Autodesk Inventor part; units mm, degrees
ref_plane "YZ Plane" through (0, 0, 0) normal (1, 0, 0) x (0, 1, 0)
ref_plane "XZ Plane" through (0, 0, 0) normal (0, 1, 0) x (-1, 0, 0)
ref_plane "XY Plane" through (0, 0, 0) normal (0, 0, 1) x (1, 0, 0)
sketch "Sketch1" plane through (0, 0, 0) normal (0, 1, 0) x (-1, 0, 0)
  circle A0 centre (0, 0) radius 57.785
  circle A1 centre (0, 0) radius 148.0058
  line L0 (0, 0) -> (-122.3635, 70.6466) construction
  line L1 (0, 0) -> (141.2932, 0) construction
  line L2 (-122.3635, 70.6466) -> (0, 0) construction
  line L3 (0, 0) -> (-128.1768, -74.0029) construction
  circle A2 centre (0, 0) radius 148.0058 construction
  line L4 (0, 0) -> (148.0058, 0) construction
  circle A3 centre (0, 0) radius 137.541 construction
  circle A4 centre (-119.114, -68.7705) radius 3.175
  circle A5 centre (0, -137.541) radius 3.175
  circle A6 centre (119.114, -68.7705) radius 3.175
  circle A7 centre (119.114, 68.7705) radius 3.175
  circle A8 centre (0, 137.541) radius 3.175
  circle A9 centre (-119.114, 68.7705) radius 3.175
  dimension "d22" = 275.082
  dimension "d16" = 115.57
  dimension "d17" = 296.0116
  dimension "d20" = 150
  dimension "d21" = 150
  dimension "d23" = 6.35
  dimension "d24" = 360
extrude "Extrusion1" add sketch "Sketch1" along normal blind 12.7
sketch "Sketch2" plane through (0, 12.7, 0) normal (0, 1, 0) x (1, 0, 0)
  circle A0 centre (0, 0) radius 123.4694 construction
  line L0 (-21.15, -84.9341) -> (-21.15, -115.9341) construction
  line L1 (15.5, -121.5841) -> (-15.5, -121.5841) construction
  line L2 (21.15, -115.9341) -> (21.15, -84.9341) construction
  line L3 (-15.5, -79.2841) -> (15.5, -79.2841) construction
  line L4 (15.5, -79.2841) -> (21.15, -84.9341) construction
  line L5 (21.15, -115.9341) -> (15.5, -121.5841) construction
  line L6 (-15.5, -121.5841) -> (-21.15, -115.9341) construction
  line L7 (-21.15, -84.9341) -> (-15.5, -79.2841) construction
  line L8 (-15.5, -115.9341) -> (15.5, -115.9341) construction
  line L9 (15.5, -115.9341) -> (15.5, -84.9341) construction
  line L10 (15.5, -84.9341) -> (-15.5, -84.9341) construction
  line L11 (-15.5, -84.9341) -> (-15.5, -115.9341) construction
  line L12 (-15.5, -115.9341) -> (15.5, -84.9341) construction
  line L13 (15.5, -115.9341) -> (-15.5, -84.9341) construction
  circle A1 centre (15.5, -84.9341) radius 1.5
  circle A2 centre (15.5, -115.9341) radius 1.5
  circle A3 centre (-15.5, -115.9341) radius 1.5
  circle A4 centre (-15.5, -84.9341) radius 1.5
  circle A5 centre (0, -100.4341) radius 11.049
  circle A6 centre (0, -100.4341) radius 22.9616 construction
  dimension "d27" = 246.9388
  dimension "d32" = 3
  dimension "d33" = 3
  dimension "d34" = 3
  dimension "d35" = 22.098
  dimension "d44" = 45.9232
extrude "Extrusion2" cut sketch "Sketch2" against normal through all
sketch "Sketch3" plane through (0, 12.7, 0) normal (0, 1, 0) x (1, 0, 0)
  line L0 (-148.0058, 50.8) -> (-148.0058, -50.8)
  line L1 (148.0058, -50.8) -> (148.0058, 50.8)
  line L2 (148.0058, 50.8) -> (-148.0058, -50.8) construction
  line L3 (-148.0058, 50.8) -> (148.0058, -50.8) construction
  line L4 (75.193, -50.8) -> (-75.193, 50.8) construction
  line L5 (-75.193, -50.8) -> (75.193, 50.8) construction
  line L6 (-148.0058, -50.8) -> (-75.193, -50.8)
  line L7 (75.193, -50.8) -> (148.0058, -50.8)
  line L8 (148.0058, 50.8) -> (75.193, 50.8)
  line L9 (-75.193, 50.8) -> (-148.0058, 50.8)
  line L10 (-75.193, -50.8) -> (-75.193, -45.7676)
  line L11 (-75.193, 45.7676) -> (-75.193, 50.8)
  line L12 (75.193, 50.8) -> (75.193, 45.7676)
  line L13 (75.193, -45.7676) -> (75.193, -50.8)
  arc A0 (75.193, -45.7676) -> (75.193, 45.7676) centre (0, 0) ccw
  arc A1 (-75.193, 45.7676) -> (-75.193, -45.7676) centre (0, 0) ccw
  dimension "d38" = 296.0116
  dimension "d39" = 101.6
extrude "Extrusion4" cut sketch "Sketch3" against normal through all
properties part number "Turntable Mount" material "PVC-Piping"
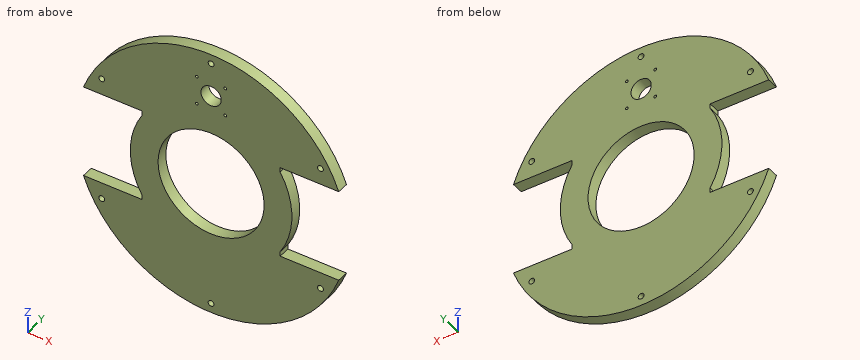
Here's how the part is built. I have some questions about the finished solid (model axes, mm). Round coordinates to 2 decimals unless told otherwise and drop trailing zeros. Write each loop counter-clockwise with the first axis right and the second up, starting at its lowest first coordinate (ties: lowest second). Pieces come first, ordered by that corner, then holes.
1. Suppose I cut it at D-D (z = -90). List the corners of the cut face in (x, y) for me.
2. I need wall thicknesses on L1, parallel to Z at x = 81.5, y = 6.5; L2, parallel to Z at x = -15.5, y = 8; L3, parallel to Z at x = -1, y = 2. Which ranges of each line are inside material? Lowest first, please.
3. Will these pins go through, and if not, where does the flat tip stop? pin 1 Ø4 at (y, z) = (6, 48.5) entering from +X; pin 2 Ø1 at (y, z) = (6.5, -10) entering from +X; pin 3 Ø4 at (x, y) = (123, 8) entering from +Z; pin 4 Ø2.5 at (x, z) = (-15.5, 84.93) entering from +Y.
4. Suppose I cut it at B-B (y = 2.75). State how many separate pieces and enclosed holes the cut face has, and give its area (3 significant figures).
5. Suppose I cut it at C-C (x = -109). List the corners of the cut face in (y, z) for me, and give its area (3 significant figures).
6. Suppose I cut it at A-A (z = 0). List the corners of the cut face in (x, y) for me (3 decimals).
Answer sheet:
1. outline: (-117.5, 0) - (117.5, 0) - (117.5, 12.7) - (-117.5, 12.7) - close
2. L1: z = -123.55 to -50.8, -33.26 to 33.26, 50.8 to 123.55
2. L2: z = -147.19 to -55.67, 55.67 to 83.43, 86.43 to 114.43, 117.43 to 147.19
2. L3: z = -148 to -140.55, -134.53 to -57.78, 57.78 to 89.43, 111.44 to 134.53, 140.55 to 148
3. pin 1: stops at x = 75.19
3. pin 2: stops at x = 87.51
3. pin 3: stops at z = 85.23
3. pin 4: passes through
4. separate pieces: 1
4. enclosed holes: 12
4. area: 45,100 mm2
5. outline: (0, -100.12) - (12.7, -100.12) - (12.7, -50.8) - (0, -50.8) - close; (0, 50.8) - (12.7, 50.8) - (12.7, 100.12) - (0, 100.12) - close
5. area: 1,250 mm2
6. outline: (-88.026, 0) - (-57.785, 0) - (-57.785, 12.7) - (-88.026, 12.7) - close; (57.785, 0) - (88.026, 0) - (88.026, 12.7) - (57.785, 12.7) - close
